Design review of the part built by this model. Coordinates are the model's own, in mm. Face numbers are marked on the shaded views. A direction names the side the tool comes from. Give positions to 0.01 mm unless a question says otherwise; leave off trailing zeros. Write each loop counter-clockwise with the first axis right and the second up, starting at its lowest first coordinate (ties: lowest second). Pieces come first, ordered by that corner, then holes. Notation, with made-up numbers: (33, 70) -> (66, 70) arc R36 cw to (66, 108) -> close; hole circle Ø5 at (56, 50). An arc over 180 degrees is marked (long way). Answer as a JSON object with one key per item and string values.
Autodesk Inventor part; units mm, degrees
ref_plane "YZ Plane" through (0, 0, 0) normal (1, 0, 0) x (0, 1, 0)
ref_plane "XZ Plane" through (0, 0, 0) normal (0, 1, 0) x (-1, 0, 0)
ref_plane "XY Plane" through (0, 0, 0) normal (0, 0, 1) x (1, 0, 0)
sketch "スケッチ1" plane through (0, 0, 0) normal (0, 0, 1) x (1, 0, 0)
  line L0 (-20, 20) -> (20, 20)
  line L1 (20, 20) -> (20, -20)
  line L2 (20, -20) -> (-20, -20)
  line L3 (-20, -20) -> (-20, 20)
  line L4 (-20, 20) -> (20, -20) construction
  line L5 (20, 20) -> (-20, -20) construction
  line L6 (-18, 18) -> (18, 18)
  line L7 (18, 18) -> (18, -18)
  line L8 (18, -18) -> (-18, -18)
  line L9 (-18, -18) -> (-18, 18)
  line L10 (-18, 18) -> (18, -18) construction
  line L11 (18, 18) -> (-18, -18) construction
  point P0 (0, 0)
  point P1 (0, 0)
  dimension "d0" = 40
  dimension "d1" = 40
  dimension "d2" = 2
  dimension "d3" = 2
extrude "押し出し1" add sketch "スケッチ1" along normal blind 83
sketch "スケッチ3" plane through (-20, 20, 0) normal (0, 1, 0) x (1, 0, 0)
  line L0 (5, -68) -> (35, -68)
  line L1 (35, -68) -> (35, -15)
  line L2 (35, -15) -> (5, -15)
  line L3 (5, -15) -> (5, -68)
  line L4 (40, -83) -> (0, -83)
  line L5 (0, 0) -> (40, 0)
  line L6 (40, 0) -> (40, -83)
  line L7 (0, 0) -> (0, -83)
  point P0 (20, 0)
  dimension "d6" = 15
  dimension "d7" = 15
  dimension "d8" = 5
  dimension "d9" = 5
extrude "押し出し2" cut sketch "スケッチ3" against normal blind 100 contours L3 L2 L1 L0
fillet "フィレット1" radius 2 8 edges at (-15, 19, 68) (-15, 19, 15) (15, 19, 15) (15, 19, 68) (15, -19, 68) (-15, -19, 68) (-15, -19, 15) (15, -19, 15)
sketch "スケッチ4" plane through (-20, 20, 0) normal (0, 1, 0) x (1, 0, 0)
  line L0 (0, 0) -> (0, -83)
  line L1 (0, 0) -> (40, 0)
  line L2 (40, 0) -> (40, -83)
  line L3 (40, -83) -> (0, -83)
  point P0 (20, 0)
  point P1 (5, -5)
  point P2 (5, -78)
  point P3 (35, -78)
  point P4 (35, -5)
  dimension "d13" = 5
  dimension "d14" = 5
  dimension "d15" = 5
  dimension "d16" = 5
  dimension "d17" = 5
  dimension "d18" = 5
  dimension "d19" = 5
  dimension "d20" = 5
hole "穴1" at (-15, 20, 5) at (-15, 20, 78) at (15, 20, 78) at (15, 20, 5) direction (0, -1, 0) diameter 2.5 end up to surface
thread "ねじ1"
thread "ねじ2"
thread "ねじ3"
thread "ねじ4"
sketch "スケッチ6" plane through (-20, -20, 0) normal (-1, 0, 0) x (0, 0, 1)
  line L0 (0, 0) -> (0, 40)
  line L1 (0, 40) -> (83, 40)
  line L2 (83, 40) -> (83, 0)
  point P0 (0, 20)
  point P1 (68, 26)
  dimension "d46" = 14
  dimension "d54" = 15
hole "穴3" at (-20, 6, 68) direction (1, 0, 0) diameter 10 depth 8
sketch "スケッチ7" plane through (-20, -20, 0) normal (-1, 0, 0) x (0, 0, 1)
  line L0 (0, 40) -> (83, 40)
  line L1 (83, 40) -> (83, 0)
  point P0 (0, 20)
  point P1 (68, 19)
  dimension "d55" = 21
  dimension "d56" = 15
hole "穴4" at (-20, -1, 68) direction (1, 0, 0) diameter 3 depth 8
pattern_circular "円形状パターン1" count 3 over 360 about axis through (-16, 6, 68) along (-1, 0, 0) of "穴4"
sketch "スケッチ8" plane through (-20, -20, 0) normal (-1, 0, 0) x (0, 0, 1)
  line L0 (83, 40) -> (83, 0)
  line L1 (0, 0) -> (83, 0)
  line L2 (0, 40) -> (83, 40)
  circle A0 centre (68, 26) radius 5
  point P0 (0, 20)
  point P1 (41.5, 26)
  dimension "d77" = 14
  dimension "d78" = 26.5
hole "穴5" at (-20, 6, 41.5) direction (1, 0, 0) diameter 6 end through all
properties part number "Gear box改" material "アルミニウム"
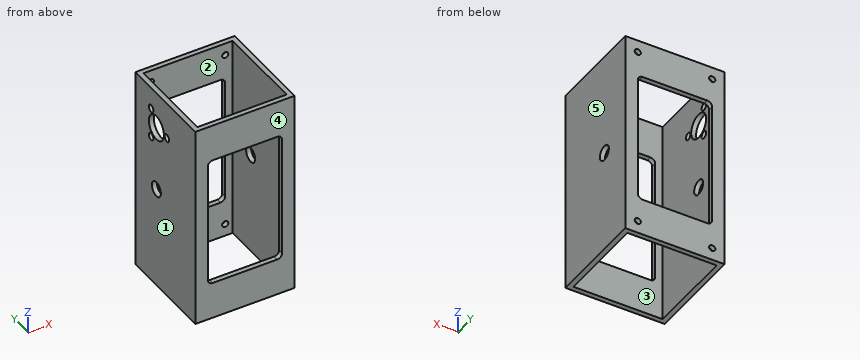
(1) Clearance check with flat-ended pins moving along their axes: pin 1 (9.5 mm diameter, centred on y = 6, z = 41.5, fed in from -X); pin 2 (2.5 mm diameter, centred on y = 9.5, z = 74.06, fed in from -X); pin 3 (12 mm diameter, centred on x = -4, z = 37.5, fed in from -Y). State where each tip first meets the part, or that it passes through.
Here are the results:
{"pin 1": "stops at x = -20", "pin 2": "stops at x = 18", "pin 3": "passes through"}
(2) We need section A-A, the plane z = 34.5. State the section outline as (x, y) points.
Here are the results:
{"outline": "(-20, -20) -> (-15, -20) -> (-15, -18) -> (-18, -18) -> (-18, 18) -> (-15, 18) -> (-15, 20) -> (-20, 20) -> close; (15, -20) -> (20, -20) -> (20, 20) -> (15, 20) -> (15, 18) -> (18, 18) -> (18, -18) -> (15, -18) -> close"}
(3) For the marked faces 1 and 2, list the 3-axis set-ups (+Z, -Z, +X, -X, +Y, -Y) from which the entire face can be reached by the end or side of a thin tool; tool diameter is ignored.
Here are the results:
{"face 1": "+Z, -Z, -X, +Y, -Y", "face 2": "+Z, -Z"}
(4) We need section D-D, the plane y = 6. State the section outline as (x, z) points, then the cut area to 3 significant figures.
Here are the results:
{"outline": "(-20, 0) -> (-18, 0) -> (-18, 38.5) -> (-20, 38.5) -> close; (-20, 44.5) -> (-18, 44.5) -> (-18, 63) -> (-20, 63) -> close; (-20, 73) -> (-18, 73) -> (-18, 83) -> (-20, 83) -> close; (18, 0) -> (20, 0) -> (20, 38.5) -> (18, 38.5) -> close; (18, 44.5) -> (20, 44.5) -> (20, 83) -> (18, 83) -> close", "area": "288 mm²"}
(5) We need section C-C, the plane y = -7. State the section outline as (x, z) points.
Here are the results:
{"outline": "(-20, 0) -> (-18, 0) -> (-18, 83) -> (-20, 83) -> close; (18, 0) -> (20, 0) -> (20, 83) -> (18, 83) -> close"}
(6) We need section B-B, the plane x = -3. State the section outline as (y, z) points, then the cut area to 3 significant figures.
Here are the results:
{"outline": "(-20, 0) -> (-18, 0) -> (-18, 15) -> (-20, 15) -> close; (-20, 68) -> (-18, 68) -> (-18, 83) -> (-20, 83) -> close; (18, 0) -> (20, 0) -> (20, 15) -> (18, 15) -> close; (18, 68) -> (20, 68) -> (20, 83) -> (18, 83) -> close", "area": "120 mm²"}
(7) For line 1 along Y through (x, z) = (-19.15, 68); line 2 along Z through (x, y) = (-19.5, 6); line 3 along X through (y, z) = (19.3, 5), list the stretches that pass through material, from the lowest coordinate up.
Here are the results:
{"line 1": "y = -20 to -2.5, 0.5 to 1, 11 to 20", "line 2": "z = 0 to 38.5, 44.5 to 63, 73 to 83", "line 3": "x = -20 to -16.25, -13.75 to 13.75, 16.25 to 20"}
(8) The part is to be moulded in two halves that separate along Y. For the marked faces 3, 4 and 5, say which applies: +Y half, -Y half, draft (parallel to the pull), parting line (faces both ways), or undercut.
Here are the results:
{"face 3": "undercut", "face 4": "-Y half", "face 5": "draft"}
